Input: part model. Units: mm. Frame: model coordinates. A direction names the side the tool comes from. Coordinates: 2 decimals unless noted, no trailing zeros. Order: outer loops, then holes, each group sorted by start corner. A loop starts at its lowest first (then second) coordinate and runs counter-clockwise, first axis right, second up. Notation, with made-up numbers: (57, -25.5) - (99, -25.5) arc R33 cw to (99, 2.5) - close; hole circle Ø8 at (57.5, -38.5). An arc over 180 degrees is marked (long way). Use a Markdown table: item, result. Add a question column.
Autodesk Inventor part; units mm, degrees
ref_plane "YZ Plane" through (0, 0, 0) normal (1, 0, 0) x (0, 1, 0)
ref_plane "XZ Plane" through (0, 0, 0) normal (0, 1, 0) x (-1, 0, 0)
sketch "Sketch5" plane through (0, 0, 0) normal (0, 0, 1) x (1, 0, 0)
  line L0 (0, 0) -> (6.35, 0)
  line L1 (6.35, 0) -> (6.35, 25.4)
  line L2 (6.35, 25.4) -> (0, 25.4)
  line L3 (0, 25.4) -> (0, 0)
  dimension "d21" = 25.4
  dimension "d22" = 6.35
extrude "Extrusion3" add sketch "Sketch5" against normal mid plane 38.1
sketch "Sketch6" plane through (0, 0, 0) normal (0, 0, 1) x (1, 0, 0)
  line L0 (6.35, 25.4) -> (6.35, 0)
  line L1 (0, 25.4) -> (6.35, 25.4)
  line L2 (6.35, 0) -> (0, 0)
  line L3 (0, 0) -> (0, 25.4)
  line L4 (6.35, 0) -> (70.8025, 23.4588)
  line L5 (6.35, 0) -> (74.9389, 0) construction
  line L6 (70.8025, 48.8588) -> (70.8025, 23.4588)
  arc A0 (37.9708, 36.909) -> (63.6292, 46.2479) centre (50.8, 41.5785) ccw
  line L7 (6.35, 25.4) -> (37.9708, 36.909)
  line L8 (63.6292, 46.2479) -> (70.8025, 48.8588)
  dimension "d25" = 20
  dimension "d26" = 27.305
  dimension "d29" = 6.35
  dimension "d30" = 50.8
  dimension "d33" = 0
extrude "Extrusion4" add sketch "Sketch6" along normal mid plane 6.35 contours L7 A0 L8 L6 L4 L0
sketch "Sketch7" plane through (6.35, 0, 19.05) normal (1, 0, 0) x (0, 0, -1)
  line L0 (38.1, 25.4) -> (0, 25.4) construction
  line L1 (6.35, 25.4) -> (6.35, 0) construction
  line L2 (31.75, 25.4) -> (31.75, 0) construction
  line L3 (0, 0) -> (0, 25.4) construction
  line L4 (38.1, 25.4) -> (38.1, 0) construction
  line L5 (0, 0) -> (15.875, 0)
  line L6 (22.225, 0) -> (38.1, 0)
  point P0 (19.05, 0)
  point P1 (6.35, 12.7)
  point P2 (31.75, 12.7)
  dimension "d34" = 6.35
  dimension "d35" = 6.35
sketch "Sketch8" plane through (0, 0, 0) normal (0, 0, 1) x (1, 0, 0)
  line L0 (0, 0) -> (0, 25.4)
  line L1 (6.35, 0) -> (0, 0)
  line L2 (70.8025, 23.4588) -> (6.35, 0)
  line L3 (0, 0) -> (6.35, 0)
  line L4 (0, -2.3112) -> (6.35, 0)
  line L5 (0, 0) -> (0, -2.3112)
extrude "Extrusion5" add sketch "Sketch8" along normal mid plane 38.1
hole "Hole3" at (6.35, 12.7, 12.7) at (6.35, 12.7, -12.7) direction (-1, 0, 0) diameter 3.81 end through all countersink diameter 7.0866 countersink angle 82
sketch "Sketch9" plane through (0, 0, 0) normal (0, 0, 1) x (1, 0, 0)
  line L0 (0, -2.3112) -> (0, 25.4)
  line L1 (0, 25.4) -> (6.35, 25.4)
  line L2 (6.35, 25.4) -> (37.9708, 36.909)
  line L3 (6.35, 25.4) -> (6.35, 0)
  line L4 (6.35, 25.4) -> (0, 25.4)
  line L5 (6.35, 25.4) -> (6.35, 0)
  line L6 (6.35, 25.4) -> (0, 23.0888)
  line L7 (0, 25.4) -> (0, 23.0888)
  point P0 (0, 0)
extrude "Extrusion6" cut sketch "Sketch9" along normal mid plane 38.1
equation "\"d21\" = supportHeight"
equation "\"d22\" = supportWidth"
equation "\"d23\" = totalScrewHoldWidth"
equation "\"d25\" = supportAngle"
equation "\"d26\" = pipeDiameter"
equation "\"d30\" = distanceFromWallToPipeCenter"
equation "\"d31\" = supportWidth"
equation "\"d47\" = totalScrewHoldWidth"
equation "\"d62\" = totalScrewHoldWidth"
equation "\"pipeDiameter\" = 27.305"
equation "\"distanceFromWallToPipeCenter\" = 50.8"
equation "\"supportHeight\" = 25.4"
equation "\"supportWidth\" = 6.35"
equation "\"screwHoldDepth\" = 6.35"
equation "\"totalScrewHoldWidth\" = 38.1"
equation "\"screwPositionFromTop\" = 6.35"
equation "\"supportAngle\" = 20deg"
properties part number "PipeSupport-2_00-020"
1) Cut plane B-B (z = 2). Return the cut outline in (x, y).
2) Contact query for flat-ended pins moving along their axis: P1, Ø14.5, axis at x = 34, y = 28, coming from the -Z side (3 decimals); P2, Ø5, axis at y = 9, z = 9.5, coming from the +X side; P3, Ø14.5, axis at x = 37.5, y = 31, coming from the +Z side (3 decimals). Output: stop coordinate, or through.
3) Reachability of faces 1 (the flat face through (6.35, 15, -9)), 2 (the flat face through (3, 12, 19.05)), 3 (the flat face through (6.35, 10, 9)) from +Z, -Z, +X, -X, +Y, -Y: full face, straight path, thin tool, end or side. Return the list, or none.
4) Material intervals for L1, parallel to Z at x = 3.45, y = 12.7 (3 decimals); L2, parallel to Z at x = 2, y = 12; L3, parallel to X at y = 12.5, z = 4, sorted ascending.
5) Cut plane A-A (z = 12.7). Return the cut outline in (x, y) (3 decimals).
6) Cut plane D-D (y = 12.7). Return the cut outline in (x, z) (3 decimals).
7) Pull-direction query (Y, two-part tool) for faces 4 (the cylindrical face through (55.75, 28.855, -0.044)), 5 (the flat face through (0, 11, 0)), 6 (the flat face through (67.166, 47.535, -0.044)); classes: pulls with the +Y half, pulls with the -Y half, needs draft (parallel to the pull), parting line crosses it, or undercut.
8) Cut plane C-C (y = 35.5). Return the cut outline in (x, z) (1 decimal), and give its area (3 significant figures).
Computed:
| question | item | result |
|---|---|---|
| 1 | outline | (0, -2.31) - (6.35, 0) - (70.8, 23.46) - (70.8, 48.86) - (63.63, 46.25) arc R13.65 cw to (37.97, 36.91) - (6.35, 25.4) - (0, 23.09) - close |
| 2 | P1 | stops at z = -3.175 |
| 2 | P2 | stops at x = 6.35 |
| 2 | P3 | stops at z = 3.175 |
| 3 | face 1 | -Z, +X, +Y, -Y |
| 3 | face 2 | +Z, +X, -X, +Y, -Y |
| 3 | face 3 | +Z, +X, +Y, -Y |
| 4 | L1 | z = -19.05 to -14.605, -10.795 to 10.795, 14.605 to 19.05 |
| 4 | L2 | z = -19.05 to -14.47, -10.93 to 10.93, 14.47 to 19.05 |
| 4 | L3 | x = 0 to 6.35 |
| 5 | outline | (0, -2.311) - (6.35, 0) - (6.35, 9.157) - (4.465, 10.795) - (0, 10.795) - close; (0, 14.605) - (4.465, 14.605) - (6.35, 16.243) - (6.35, 25.4) - (0, 23.089) - close |
| 6 | outline | (0, -19.05) - (6.35, -19.05) - (6.35, -16.243) - (4.465, -14.605) - (0, -14.605) - close; (0, -10.795) - (4.465, -10.795) - (6.35, -9.157) - (6.35, -3.175) - (41.243, -3.175) - (41.243, 3.175) - (6.35, 3.175) - (6.35, 9.157) - (4.465, 10.795) - (0, 10.795) - close; (0, 14.605) - (4.465, 14.605) - (6.35, 16.243) - (6.35, 19.05) - (0, 19.05) - close |
| 7 | face 4 | undercut |
| 7 | face 5 | needs draft |
| 7 | face 6 | pulls with the +Y half |
| 8 | outline | (34.1, -3.2) - (38.6, -3.2) - (38.6, 3.2) - (34.1, 3.2) - close; (63, -3.2) - (70.8, -3.2) - (70.8, 3.2) - (63, 3.2) - close |
| 8 | area | 77.8 mm2 |
